Autodesk Inventor part; units mm, degrees
ref_plane "YZ Plane" through (0, 0, 0) normal (1, 0, 0) x (0, 1, 0)
ref_plane "XZ Plane" through (0, 0, 0) normal (0, 1, 0) x (-1, 0, 0)
ref_plane "XY Plane" through (0, 0, 0) normal (0, 0, 1) x (1, 0, 0)
sketch "Sketch1" plane through (0, 0, 0) normal (0, 0, 1) x (1, 0, 0)
  line L0 (0, 0) -> (25.4, 0)
  line L1 (25.4, 0) -> (25.4, 1.5875)
  line L2 (1.5875, 25.4) -> (0, 25.4)
  line L3 (0, 25.4) -> (0, 0)
  line L4 (1.5875, 25.4) -> (1.5875, 1.5875)
  line L5 (1.5875, 1.5875) -> (25.4, 1.5875)
  dimension "d0" = 25.4
  dimension "d1" = 25.4
  dimension "d2" = 1.5875
  dimension "d3" = 1.5875
extrude "Extrusion1" add sketch "Sketch1" along normal blind 304.8
sketch "Sketch3" plane through (0, 0, 0) normal (-1, 0, 0) x (0, 0, 1)
  line L0 (304.8, 0) -> (304.8, 25.4)
  line L1 (0, 25.4) -> (304.8, 25.4)
  line L2 (0, 0) -> (304.8, 0)
  circle A0 centre (298.45, 19.05) radius 1.5875
  circle A1 centre (285.75, 7.9375) radius 1.5875
  line L3 (152.4, 25.4) -> (152.4, 0) construction
  circle A2 centre (6.35, 19.05) radius 1.5875
  circle A3 centre (19.05, 7.9375) radius 1.5875
  dimension "d19" = 6.35
  dimension "d20" = 6.35
  dimension "d21" = 7.9375
  dimension "d22" = 19.05
  dimension "d23" = 3.175
extrude "Extrusion4" cut sketch "Sketch3" against normal blind 25.4
equation "\"d2\" = d3"
equation "\"d20\" = d19"
properties part number "8 ball front L"
The listing builds one solid part. Answer for the finished solid, in the listing's coordinates (mm). A direction names the side the tool comes from. Coordinates: 2 decimals unless noted, no trailing zeros. Loops run counter-clockwise (first coordinate to the right, second up) from the corner with the lowest first, then second, coordinate; pieces in that order, holes last. Notation, with made-up numbers: M 46.5,88 L 96.5,88 A10 cw 96.5,104 Z; hole C 14,-11 d1. An arc over 180 degrees is marked long. Answer as CSV lines item,"result". Start each with the question number.
(1) For faces 1 (the flat face through (13, 0, 150)), 2 (the flat face through (13, 1.588, 150)), determine the directions among +Z, -Z, +X, -X, +Y, -Y from which every point of the face is accessible in a straight line to the end or side of a thin tool.
(2) Find the intervals of material crossed by L1, parallel to Y at x = 1.15, z = 285.75 (3 decimals); L2, parallel to X at y = 12.5, z = 81, in increasing order. Write a range as [from, to].
(3) The part is cut by section B-B (x = 22). Give the vertices of the cut face in (y, z).
(4) The part is cut by section A-A (z = 148). Give the vertices of the cut face in (x, y).
(5) Given pin 1 (3 mm diameter, centred on y = 7.94, z = 285.75, fed in from -X); pin 2 (5 mm diameter, centred on y = 19.05, z = 6.35, fed in from +X); pin 3 (2 mm diameter, centred on x = 19, z = 78, fed in from +Y), each flat-ended and moving along its own axis, determine where each tip first touches the part or whether it passes through.
Determined:
1,face 1,"+Z, -Z, +X, -X, -Y"
1,face 2,"+Z, -Z, +X, +Y"
2,L1,"[0, 6.35], [9.525, 25.4]"
2,L2,"[0, 1.59]"
3,outline,"M 0,0 L 1.59,0 L 1.59,304.8 L 0,304.8 Z"
4,outline,"M 0,0 L 25.4,0 L 25.4,1.59 L 1.59,1.59 L 1.59,25.4 L 0,25.4 Z"
5,pin 1,"through"
5,pin 2,"x = 1.59"
5,pin 3,"y = 1.59"
